from build123d import *

# Parameters (mm, degrees)
F2_R     = 7.848918
F3_DEPTH = 25
F4_R     = 10
F5_SIZE  = 5
F6_SIZE  = 5
F7_SIZE  = 2


with BuildPart() as f1:
    # F0 (on Front) → F1 (revolve)
    with BuildSketch(Plane.XZ):
        Polygon((-16.244069, 62.022675), (-22.966566, 62.022675), (-22.966566, 75.819135), (-39.015342, 75.819135), (-39.015342, 62.022675), (-39.015342, 44.167664), (-18.230908, 44.167664), (-18.230908, 21.613961), (-33.250585, 21.613961), (-33.250585, 8.26969), (16.53938, 8.26969), (16.53938, 21.613961), (0, 21.613961), (0, 44.167664), (29.707231, 44.167664), (29.707231, 62.022675), (29.707231, 75.067952), (19.069998, 75.067952), (19.069998, 62.022675), (12.920965, 62.022675), (12.920965, 64.699598), (11.734917, 64.699598), (11.734917, 78.378163), (10.245941, 78.378163), (10.245941, 64.699598), (8.93096, 64.699598), (8.93096, 62.022675), (5.415956, 62.022675), (5.415956, 64.699598), (3.918254, 64.699598), (3.918254, 78.378163), (2.611384, 78.378163), (2.611384, 64.699598), (0, 64.699598), (0, 62.022675), (-3.609054, 62.022675), (-3.609054, 64.699598), (-4.979474, 64.699598), (-4.979474, 78.378163), (-6.571971, 78.378163), (-6.571971, 64.699598), (-9.30906, 64.699598), (-9.30906, 62.022675), (-11.874064, 62.022675), (-11.874064, 64.699598), (-13.187167, 64.699598), (-13.187167, 78.378163), (-14.52281, 78.378163), (-14.52281, 64.699598), (-16.244069, 64.699598), align=None)
    revolve(axis=Axis((13.626195, 0, 0), (1, 0, 0)))

    # F2 (on face) → F3 (cut)
    with BuildSketch(Plane.YZ):
        with Locations((0, 31.763129)):
            Circle(F2_R)
        with Locations((30.208531, 9.815347)):
            Circle(F2_R)
        with Locations((18.669899, -25.696911)):
            Circle(F2_R)
        with Locations((-18.669899, -25.696911)):
            Circle(F2_R)
        with Locations((-30.208531, 9.815347)):
            Circle(F2_R)
    extrude(amount=-F3_DEPTH, mode=Mode.SUBTRACT)

    # F4
    f4_edges = [f1.edges().sort_by_distance(p)[0] for p in [
        (-39.015342, 0, -44.167664),
        (29.707231, 0, -44.167664),
    ]]
    fillet(f4_edges, radius=F4_R)

    # F5
    f5_edges = [f1.edges().sort_by_distance(p)[0] for p in [
        (16.53938, 0, -21.613961),
        (-33.250585, 0, -21.613961),
    ]]
    chamfer(f5_edges, length=F5_SIZE)

    # F6
    f6_edges = [f1.edges().sort_by_distance(p)[0] for p in [
        (16.53938, 0, -8.26969),
        (-33.250585, 0, -8.26969),
    ]]
    chamfer(f6_edges, length=F6_SIZE)

    # F7
    f7_edges = [f1.edges().sort_by_distance(p)[0] for p in [
        (0, -7.848918, 31.763129),
        (0, 22.359612, 9.815347),
        (0, 10.82098, -25.696911),
        (0, -26.518817, -25.696911),
        (0, -38.057449, 9.815347),
        (-18.230908, -7.848918, 31.763129),
        (-18.230908, -38.057449, 9.815347),
        (-18.230908, -26.518817, -25.696911),
        (-18.230908, 10.82098, -25.696911),
        (-18.230908, 22.359612, 9.815347),
    ]]
    chamfer(f7_edges, length=F7_SIZE)


solid = f1.part
Build history of the part. All positions in model axes, mm. A direction names the side the tool comes from. Give positions to 0.01 mm unless a question says otherwise; leave off trailing zeros. Order: outer loops, then holes, each group sorted by start corner. A loop starts at its lowest first (then second) coordinate and runs counter-clockwise, first axis right, second up. Notation, with made-up numbers: M -22,2.5 L 27,2.5 A24 cw 27,39.5 Z; hole C 9.25,35 d11. An arc over 180 degrees is marked long. Use one line per item in the form item = value.
Q1. Pull direction X, two halves, no side cores. Call faces 3 (the flat face through (-14.523, -64, 11)), 4 (the cylindrical face through (9.99, 43.12, -9.57)), 5 (the flat face through (-33.251, 13.5, -1.3)): released by +X, released by -X, zero draft, split by the parting line, or undercut.
Conclusion:
face_3 = undercut
face_4 = zero draft
face_5 = released by -X
Q2. Wall check: probe 1 along Z at (x, y) = (-11, 0); probe 2 along X at (y, z) = (54, -31); probe 3 along Y at (x, z) = (-20.5, 0). Give the ranges that are in metal, low to high.
Conclusion:
probe_1 = -62.02 to -8.27, 8.27 to 23.91, 39.61 to 62.02
probe_2 = -39.02 to -22.97, -16.24 to -11.87, -9.31 to -3.61, 0 to 5.42, 8.93 to 12.92, 19.07 to 29.71
probe_3 = -62.02 to -44.17, -21.61 to -8.27, 8.27 to 21.61, 44.17 to 62.02
Q3. Pin check, flat tips, straight feed: P1, Ø1, axis at x = 6.5, z = 51, coming from the +Y side; P2, Ø12, axis at y = -14.5, z = -29.5, coming from the +X side; P3, Ø12, axis at x = -20.5, z = 54, coming from the -Y side. Stop position of each tip, or through.
Conclusion:
P1 = 36.01
P2 = 0
P3 = -58.25
Q4. Slice it at D-D, the plane x = 25.5. Write the cut outline in (y, z).
Conclusion:
outline = C 0,0 d150.14; hole C 0,0 d92.03
Q5. Slice it at B-B, the plane z = 67. Write the cut outline in (x, y), and give its area (4 significant figures).
Conclusion:
outline = M -39.02,-35.49 L -22.97,-35.49 L -22.97,35.49 L -39.02,35.49 Z; M -14.52,-40.67 L -13.19,-40.67 L -13.19,40.67 L -14.52,40.67 Z; M -6.57,-40.67 L -4.98,-40.67 L -4.98,40.67 L -6.57,40.67 Z; M 2.61,-40.67 L 3.92,-40.67 L 3.92,40.67 L 2.61,40.67 Z; M 10.25,-40.67 L 11.73,-40.67 L 11.73,40.67 L 10.25,40.67 Z; M 19.07,-33.86 L 29.71,-33.86 L 29.71,33.86 L 19.07,33.86 Z
area = 2,325 mm2
Q6. Which spindle directions (+Z, -Z, +X, -X, +Y, -Y) get a long thin tool onto all of the face, cutting with end or side? Do faces 1 (the cylindrical face through (-9.02, -20.37, -33.36)), 2 (the flat face through (19.07, -56, -28)). Say none if no direction does.
Conclusion:
face_1 = +X, -X
face_2 = none
Q7. Slice it at A-A, the plane x = -26. Write the cut outline in (y, z), and give its area (3 significant figures).
Conclusion:
outline = C 0,0 d151.64; C 0,0 d43.23; hole C 0,0 d88.34; hole C 0,0 d16.54
area = 13,200 mm2
Q8. Slice it at C-C, the plane y = 0. State how many separate pieces and enclosed holes the cut face has, and give its area (3 significant figures).
Conclusion:
separate_pieces = 3
enclosed_holes = 0
area = 5,110 mm2
